```python
from build123d import *

# Parameters (mm, degrees)
CUT_EXTRUDE1_DEPTH = 30
CHAMFER1_SIZE      = 1
CHAMFER2_SIZE      = 1


with BuildPart() as part:
    # Sketch1 → Revolve1 (revolve)
    with BuildSketch(Plane.XY, mode=Mode.PRIVATE) as revolve1_sk:
        Polygon((15, 15), (15, 25.344902759), (2.5, 26), (2.5, 60), (8.480762114, 60), (12.5, 75), (7.323619098, 75), (4.644127174, 65), (-4.644127174, 65), (-7.323619098, 75), (-12.5, 75), (-8.480762114, 60), (-2.5, 60), (-2.5, 26), (-15, 25.344902759), (-15, 15), align=None)
    revolve(revolve1_sk.sketch.rotate(Axis((0, 0, 0), (1, 0, 0)), 90), axis=Axis((0, 0, 0), (1, 0, 0)))

    # Sketch2 → Cut-Extrude1 (cut)
    with BuildSketch(Plane(origin=(15, 0, 0), x_dir=(0, 0, -1), z_dir=(1, 0, 0))):
        with BuildLine():
            Line((-14.585952146, 3.5), (-17.5, 3.5))
            Line((-17.5, 3.5), (-17.5, -3.5))
            Line((-17.5, -3.5), (-14.585952146, -3.5))
            ThreePointArc((-14.585952146, -3.5), (15, 0), (-14.585952146, 3.5))
        make_face()
    extrude(amount=-CUT_EXTRUDE1_DEPTH, mode=Mode.SUBTRACT)

    # Chamfer1
    chamfer1_edges = [part.edges().sort_by_distance(p)[0] for p in [
        (15, 0, -15),
    ]]
    chamfer(chamfer1_edges, length=CHAMFER1_SIZE)

    # Chamfer2
    chamfer2_edges = [part.edges().sort_by_distance(p)[0] for p in [
        (-15, 0, -15),
    ]]
    chamfer(chamfer2_edges, length=CHAMFER2_SIZE)


solid = part.part
```
The model under review builds one solid part; all positions refer to its coordinate system, in mm. A direction names the side the tool comes from. Round coordinates to 2 decimals unless told otherwise and drop trailing zeros. Use CSV: the item, a comma, the result in double quotes. Start each with the question number.
(1) For line 1 along Z through (x, y) = (-4, -3); line 2 along Y through (x, z) = (4.45, 0); line 3 along Z through (x, y) = (3.25, 12), list the stretches that pass through material, from the lowest coordinate up.
(2) The part is to be moulded in two halves that separate along Y. For faces 1 (the face through (-0.07, -19.52, 62)), 2 (the face through (8.73, -18.3, 58.12)), 3 (the face through (15, 0, -17)), say which applies: +Y half, -Y half, draft (parallel to the pull), parting line (faces both ways), or undercut.
(3) Tool access review of faces 4 (the face through (2.5, 12, -26)), 5 (the face through (4.774, -19.67, 62.462)), 6 (the face through (-2.5, 26, 12)): name each direction out of +Z, -Z, +X, -X, +Y, -Y from which nothing blocks a thin tool from reaching the whole face with its end or side.
(4) Clearance check with flat-ended pins moving along their axes: P1, Ø12, axis at y = -50, z = 47.5, coming from the +X side; P2, Ø6, axis at y = 37.5, z = 13, coming from the -X side; P3, Ø6, axis at x = 10, y = -47.5, coming from the -Z side. State where each tip first meets the part, or that it passes through.
Findings:
1,line 1,"-64.93 to -59.92, -25.75 to -14.7, 17.5 to 25.75, 59.92 to 64.93"
1,line 2,"-65 to -60, -25.9 to -15, 15 to 25.9, 60 to 65"
1,line 3,"-63.88 to -58.79, -23.02 to -9, 9 to 23.02, 58.79 to 63.88"
2,face 1,"parting line"
2,face 2,"undercut"
2,face 3,"draft"
3,face 4,"+X"
3,face 5,"none"
3,face 6,"-X"
4,P1,"x = 12.49"
4,P2,"x = -2.5"
4,P3,"z = -60.37"
